Could you check a few things on this model? Use its own coordinates, in mm. A direction names the side the tool comes from. Give positions to 0.01 mm unless a question says otherwise; leave off trailing zeros. Loops run counter-clockwise (first coordinate to the right, second up) from the corner with the lowest first, then second, coordinate; pieces in that order, holes last. Notation, with made-up numbers: M 84,55.25 L 133,55.25 A12 ccw 133,72.25 Z; hole C -25,14.5 d9. An arc over 180 degrees is marked long. Use a Markdown table: item, result. Add a question column.
1) Suppose I cut it at C-C on y = 8. List the corners of the cut face in (x, z) for me.
2) If I drill on line 1 along Z through (x, y) = (0, 18.75); line 2 along X through (y, z) = (-45.5, -2.25), over which ranges is the centre line in solid material (lowest first)? Write a range as [from, to].
3) Suppose I cut it at A-A on z = 0. List the corners of the cut face in (x, y) for me.
4) Suppose I cut it at D-D on z = -3.75. List the corners of the cut face in (x, y) for me, and give its area (3 significant figures).
5) Suppose I cut it at B-B on x = 0. List the corners of the cut face in (y, z) for me, and give its area (3 significant figures).
6) Will these pins go through, and if not, where does the flat tip stop? pin 1 Ø5 at (y, z) = (-27.5, 4) entering from -X; pin 2 Ø1.5 at (x, y) = (2, -36.5) entering from +Z; pin 3 Ø4.5 at (x, y) = (0.5, -32.5) entering from -Z; pin 4 Ø2.5 at (x, z) = (5.5, -6) entering from +Y.
7) We'd pull the mould along Z, two halves only. Please class faces 1 (the flat face through (0, -39, -7.5)), 2 (the flat face through (0, 11, 0)), 3 (the flat face through (-7.5, -39, 0)): +Z half, -Z half, draft (parallel to the pull), parting line (faces both ways), or undercut.
8) Which directions (+Z, -Z, +X, -X, +Y, -Y) give clear straight access to the entire face, cutting with the end or side of a thin tool? Please do faces 4 (the flat face through (7.5, -39, 0)), 5 (the flat face through (6, 0, -6)), 6 (the cylindrical face through (-1.73, 10.85, 7.81)).
```python
from build123d import *

# Parameters (mm, degrees)
SKETCH_1_R          = 8
EXTRUDE_1_DEPTH     = 22
SKETCH_2_W          = 15
SKETCH_2_H          = 15
EXTRUDE_2_DEPTH     = 80
SKETCH_3_R          = 2
CUT_EXTRUDE_1_DEPTH = 11


with BuildPart() as part:
    # 草图1 → 凸台-拉伸1 (new body)
    with BuildSketch(Plane(origin=(0, 0, 0), x_dir=(1, 0, 0), z_dir=(0, 1, 0))):
        Circle(SKETCH_1_R)
    extrude(amount=EXTRUDE_1_DEPTH)

    # 草图2 → 凸台-拉伸2 (add)
    with BuildSketch(Plane.XZ):
        Rectangle(SKETCH_2_W, SKETCH_2_H)
    extrude(amount=EXTRUDE_2_DEPTH)

    # 草图3 → 切除-拉伸1 (cut)
    with BuildSketch(Plane(origin=(0, 22, 0), x_dir=(1, 0, 0), z_dir=(0, 1, 0))):
        Circle(SKETCH_3_R)
    extrude(amount=-CUT_EXTRUDE_1_DEPTH, mode=Mode.SUBTRACT)


solid = part.part
```
Answer block:
| question | item | result |
|---|---|---|
| 1 | outline | C 0,0 d16 |
| 2 | line 1 | z = [-8, -2], [2, 8] |
| 2 | line 2 | x = [-7.5, 7.5] |
| 3 | outline | M -8,0 L -7.5,0 L -7.5,-80 L 7.5,-80 L 7.5,0 L 8,0 L 8,22 L 2,22 L 2,11 L -2,11 L -2,22 L -8,22 Z |
| 4 | outline | M -7.5,-80 L 7.5,-80 L 7.5,0 L 7.07,0 L 7.07,22 L -7.07,22 L -7.07,0 L -7.5,0 Z |
| 4 | area | 1,510 mm^2 |
| 5 | outline | M -80,-7.5 L 0,-7.5 L 0,-8 L 22,-8 L 22,-2 L 11,-2 L 11,2 L 22,2 L 22,8 L 0,8 L 0,7.5 L -80,7.5 Z |
| 5 | area | 1,510 mm^2 |
| 6 | pin 1 | stops at x = -7.5 |
| 6 | pin 2 | stops at z = 7.5 |
| 6 | pin 3 | stops at z = -7.5 |
| 6 | pin 4 | stops at y = 22 |
| 7 | face 1 | -Z half |
| 7 | face 2 | undercut |
| 7 | face 3 | draft |
| 8 | face 4 | +Z, -Z, +X, -Y |
| 8 | face 5 | -Z, +X, +Y |
| 8 | face 6 | +Y |
